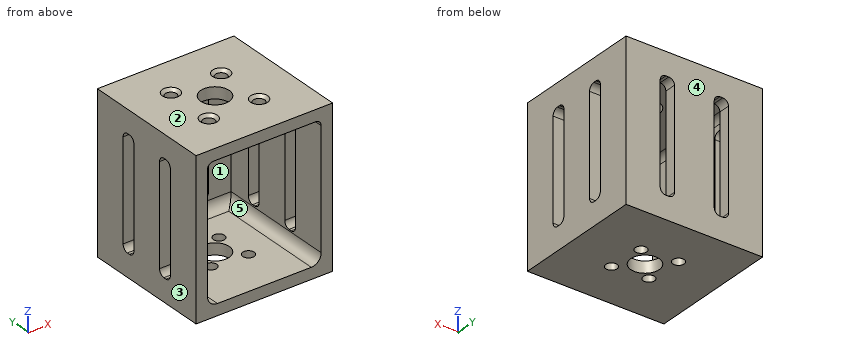
Autodesk Fusion 360 part; units mm, degrees
sketch "Sketch1" plane through (0, 0, 0) normal (0, 0, 1) x (1, 0, 0)
  line L0 (-24, -23) -> (24, -23)
  line L1 (24, -23) -> (24, 23)
  line L2 (24, 23) -> (-24, 23)
  line L3 (-24, 23) -> (-24, -23)
  dimension "d1" = 48
  dimension "d2" = 46
  dimension "d3" = 24
  dimension "d4" = 23
extrude "Extrude1" add sketch "Sketch1" along normal blind 55
sketch "Sketch2" plane through (0, -23, 0) normal (0, -1, 0) x (1, 0, 0)
  line L0 (-24, 0) -> (24, 0)
  line L1 (24, 0) -> (24, 55)
  line L2 (24, 55) -> (-24, 55)
  line L3 (-24, 55) -> (-24, 0)
  line L4 (-20, 51) -> (20, 51)
  line L5 (20, 51) -> (20, 4)
  line L6 (20, 4) -> (-20, 4)
  line L7 (-20, 4) -> (-20, 51)
  dimension "d7" = 40
  dimension "d8" = 20
  dimension "d10" = 4
  dimension "d58" = 4
extrude "Extrude2" cut sketch "Sketch2" against normal blind 42 contours L4 L5 L6 L7
sketch "Sketch4" plane through (0, 0, 55) normal (0, 0, 1) x (-1, 0, 0)
  line L0 (24, -23) -> (24, 23)
  line L1 (24, 23) -> (-24, 23)
  line L2 (-24, 23) -> (-24, -23)
  line L3 (-24, -23) -> (24, -23)
  circle A0 centre (0, 0) radius 5
  dimension "d23" = 10
hole "Hole1" at (0, 0, 55) direction (0, 0, -1) diameter 10 depth 4 tip angle 118
sketch "Sketch5" plane through (0, 0, 55) normal (0, 0, 1) x (-1, 0, 0)
  circle A0 centre (0, 0) radius 5
  line L0 (24, -23) -> (24, 23)
  line L1 (24, 23) -> (-24, 23)
  line L2 (-24, 23) -> (-24, -23)
  line L3 (-24, -23) -> (24, -23)
  circle A1 centre (-8.8388, -8.8388) radius 1.5
  point P0 (8.8388, -8.8388)
  point P1 (8.8388, 8.8388)
  point P2 (-8.8388, 8.8388)
  dimension "d27" = 12.5
  dimension "d28" = 3
  dimension "d30" = 360
hole "Hole2" at (8.8388, 8.8388, 55) at (-8.8388, 8.8388, 55) at (-8.8388, -8.8388, 55) at (8.8388, -8.8388, 55) direction (0, 0, -1) diameter 4 depth 4 tip angle 118 countersink diameter 6 countersink angle 90
sketch "Sketch7" plane through (0, 0, 0) normal (0, 0, -1) x (1, 0, 0)
  line L0 (-24, 23) -> (-24, -23)
  line L1 (-24, -23) -> (24, -23)
  line L2 (24, -23) -> (24, 23)
  line L3 (24, 23) -> (-24, 23)
  circle A0 centre (0, 0) radius 5
  circle A1 centre (5.6569, -5.6569) radius 2
  circle A2 centre (6.7175, 6.7175) radius 2
  circle A3 centre (-6.7175, -6.7175) radius 2
  circle A4 centre (-5.6569, 5.6569) radius 2
  dimension "d45" = 10
  dimension "d67" = 4
  dimension "d68" = 4
  dimension "d69" = 9.5
  dimension "d70" = 8
  dimension "d71" = 17.3431
  dimension "d72" = 16.2825
  dimension "d74" = 360
extrude "Extrude4" cut sketch "Sketch7" against normal blind 4 contours A0 | A1 | A2 | A3 | A4
sketch "Sketch8" plane through (0, 0, 55) normal (0, 0, 1) x (-1, 0, 0)
  circle A0 centre (0, 0) radius 5
  line L0 (24, -23) -> (24, 23)
  line L1 (24, 23) -> (-24, 23)
  line L2 (-24, 23) -> (-24, -23)
  line L3 (-24, -23) -> (24, -23)
  ellipse E0 centre (0, 0) end of major axis (0, 8.5421) minor radius 3.3168
  line L4 (0, -8.5421) -> (0, 8.5421)
  line L5 (3.3168, 0) -> (-3.3168, 0)
  circle A1 centre (8.8388, 8.8388) radius 3
  circle A2 centre (-8.8388, -8.8388) radius 3
  circle A3 centre (8.8388, -8.8388) radius 3
  circle A4 centre (-8.8388, 8.8388) radius 3
extrude "Extrude5" cut sketch "Sketch8" against normal blind 4 contours A0 E0 | A0 E0
sketch "Sketch3" plane through (24, 0, 0) normal (1, 0, 0) x (0, 1, 0)
  line L0 (-21, 0) -> (23, 0)
  line L1 (23, 0) -> (23, 50)
  line L2 (23, 50) -> (-21, 50)
  line L3 (-11, 47) -> (-6, 47)
  line L4 (-6, 47) -> (-6, 8)
  line L5 (-6, 8) -> (-11, 8)
  line L6 (-11, 8) -> (-11, 47)
  line L7 (6, 47) -> (11, 47)
  line L8 (11, 47) -> (11, 8)
  line L9 (11, 8) -> (6, 8)
  line L10 (6, 8) -> (6, 47)
  line L11 (-23, 0) -> (23, 0)
  line L12 (23, 0) -> (23, 55)
  line L13 (23, 55) -> (-23, 55)
  line L14 (-23, 55) -> (-23, 0)
  line L15 (-23, 51) -> (-23, 4)
  point P0 (-23, 55)
  point P1 (23, 55)
  dimension "d16" = 8
  dimension "d20" = 12
  dimension "d60" = 8
  dimension "d75" = 5
  dimension "d76" = 5
  dimension "d97" = 12
  dimension "d100" = 8
  dimension "d101" = 8
extrude "Extrude6" cut sketch "Sketch3" against normal blind 48 contours L3 L4 L5 L6 | L7 L8 L9 L10
sketch "Sketch9" plane through (0, 23, 0) normal (0, 1, 0) x (-1, 0, 0)
  line L0 (-24, 0) -> (24, 0)
  line L1 (24, 0) -> (24, 55)
  line L2 (24, 55) -> (-24, 55)
  line L3 (-24, 55) -> (-24, 0)
  line L4 (-12, 47) -> (-7, 47)
  line L5 (-7, 47) -> (-7, 8)
  line L6 (-7, 8) -> (-12, 8)
  line L7 (-12, 8) -> (-12, 47)
  line L8 (7, 47) -> (12, 47)
  line L9 (12, 47) -> (12, 8)
  line L10 (12, 8) -> (7, 8)
  line L11 (7, 8) -> (7, 47)
  line L12 (-24, 0) -> (24, 0)
  dimension "d79" = 8
  dimension "d80" = 8
  dimension "d81" = 8
  dimension "d82" = 8
  dimension "d83" = 12
  dimension "d84" = 12
  dimension "d85" = 5
  dimension "d86" = 5
extrude "Extrude7" cut sketch "Sketch9" against normal blind 44 contours L4 L5 L6 L7 | L8 L9 L10 L11
fillet "Fillet2" radius 3.5 3 edges at (0, 19, 4) (-20, -2, 4) (20, -2, 4)
fillet "Fillet3" radius 2 24 edges at (22, 11, 8) (22, -6, 8) (-22, 11, 8) (-22, -6, 8) (22, 6, 8) (22, -11, 8) (22, -11, 47) (22, 6, 47) (22, 11, 47) (22, -6, 47) (-22, -6, 47) (-22, -11, 47) (-22, 6, 47) (-22, 11, 47) (-22, -11, 8) (-22, 6, 8) (-7, 21, 8) (12, 21, 8) (7, 21, 8) (-12, 21, 8) (12, 21, 47) (-7, 21, 47) (7, 21, 47) (-12, 21, 47)
fillet "Fillet4" radius 2 3 edges at (-20, -2, 51) (0, 19, 51) (20, -2, 51)
Design review of the part built by this model. Coordinates are the model's own, in mm. Face numbers are marked on the shaded views. A direction names the side the tool comes from. Round coordinates to 2 decimals unless told otherwise and drop trailing zeros. Write each loop counter-clockwise with the first axis right and the second up, starting at its lowest first coordinate (ties: lowest second). Pieces come first, ordered by that corner, then holes. Notation, with made-up numbers: (-40, 81) - (-16, 81) arc R29 ccw to (-16, 120) - close; hole circle Ø2 at (66, 35). An arc over 180 degrees is marked (long way). Return JSON: item names as keys, results as strings. Group by question number.
Item 1: Insertion check: P1, Ø1.5, axis at x = -5.5, z = 14.5, coming from the -Y side; P2, Ø2.5, axis at x = -8.84, y = -8.84, coming from the +Z side. Each pin has a flat end and moves straight along its axis. Give the tip position at first contact, or say it passes through.
Item 2: We need section C-C on y = 0. Write out the cut boundary in (x, z), and give its area (3 significant figures).
Item 3: For probe 1 along Y at (x, z) = (21, 17); probe 2 along X at (y, z) = (20, 19); probe 3 along Z at (x, y) = (-8, -17), list the stretches that pass through material, from the lowest coordinate up. Write a range as [from, to].
Item 4: Machinability: for the marked faces 1 and 2, which of the approach directions +Z, -Z, +X, -X, +Y, -Y give a long, thin tool a straight path to every point of the face, cutting with its end or side? Answer none if there is none.
Item 5: The part is to be moulded in two halves that separate along X. For the marked faces 3, 4 and 5, say which applies: pulls with the +X half, pulls with the -X half, needs draft (parallel to the pull), parting line crosses it, or undercut.
Item 6: We need section D-D on x = -14. Write out the cut boundary in (y, z).
Item 7: We need section A-A on z = 30. Give the number of separate pieces and of enclosed holes in the cut face, and give its area (3 significant figures).
Item 8: We need section B-B on x = 0. Write out the cut boundary in (y, z).
Model answer:
{
 "1": {"P1": "stops at y = 19", "P2": "stops at z = 4"},
 "2": {"outline": "(-24, 0) - (-5, 0) - (-5, 4) - (-16.5, 4) arc R3.5 cw to (-20, 7.5) - (-20, 49) arc R2 cw to (-18, 51) - (-5, 51) - (-5, 55) - (-24, 55) - close; (5, 0) - (24, 0) - (24, 55) - (5, 55) - (5, 51) - (18, 51) arc R2 cw to (20, 49) - (20, 7.5) arc R3.5 cw to (16.5, 4) - (5, 4) - close", "area": "687 mm²"},
 "3": {"probe 1": "y = [-23, -11], [-6, 6], [11, 23]", "probe 2": "x = [-24, -12], [-7, 7], [12, 24]", "probe 3": "z = [0, 4], [51, 55]"},
 "4": {"face 1": "-Y", "face 2": "+Z, +X, -X, +Y, -Y"},
 "5": {"face 3": "pulls with the -X half", "face 4": "needs draft", "face 5": "undercut"},
 "6": {"outline": "(-23, 0) - (23, 0) - (23, 55) - (-23, 55) - (-23, 51) - (17, 51) arc R2 cw to (19, 49) - (19, 7.5) arc R3.5 cw to (15.5, 4) - (-23, 4) - close"},
 "7": {"separate pieces": "7", "enclosed holes": "0", "area": "408 mm²"},
 "8": {"outline": "(-23, 0) - (-5, 0) - (-5, 4) - (-23, 4) - close; (-23, 51) - (-5, 51) - (-5, 55) - (-23, 55) - close; (5, 0) - (23, 0) - (23, 55) - (5, 55) - (5, 51) - (17, 51) arc R2 cw to (19, 49) - (19, 7.5) arc R3.5 cw to (15.5, 4) - (5, 4) - close"}
}
